Verification items for the finished model (mm, model axes). A direction names the side the tool comes from. Coordinates: 2 decimals unless noted, no trailing zeros. Order: outer loops, then holes, each group sorted by start corner. A loop starts at its lowest first (then second) coordinate and runs counter-clockwise, first axis right, second up. Notation, with made-up numbers: M -21.5,-10 L -9.5,-10 A24 cw -9.5,7 Z; hole C -30,64 d9. An arc over 180 degrees is marked long. Return JSON: item names as keys, results as strings. Group by question number.
Q1. Go/stop test with flat-tipped pins: pin 1 Ø6 at (x, z) = (4, 2.5) entering from -Y; pin 2 Ø6 at (y, z) = (68, -0.5) entering from +X (3 decimals); pin 3 Ø4 at (x, y) = (-4.5, 101) entering from +Z; pin 4 Ø2 at (y, z) = (44, 3.5) entering from +X. Record where each tip stops, or that it passes through.
Q2. Thickness scan on probe 1 along Y at (x, z) = (4.5, 1.5); probe 2 along Z at (x, y) = (0.25, 40). Record the ranges inside material, lowest first.
Q3. Section check A-A, the plane x = 0. Enter the section's corners in (y, z) (3 decimals), then the cut area to 3 significant figures.
Q4. Section check B-B, the plane y = 171. Enter the section's corners in (x, z) (3 decimals), then the cut area to 3 significant figures.
Q5. Access from +Z, -Z, +X, -X, +Y, -Y to the whole of each face (thin tool, end or side, straight path). Record for faces 1 (the face through (0, 2, 5.556)), 2 (the face through (3, 4.366, -3)).
from build123d import *

# Parameters (mm, degrees)
BOSS_EXTRUDE1_DEPTH = 4.365625
SKETCH2_R           = 3.175
BOSS_EXTRUDE2_DEPTH = 177.8


with BuildPart() as part:
    # Sketch1 → Boss-Extrude1 (new body)
    with BuildSketch(Plane(origin=(0, 0, 0), x_dir=(1, 0, 0), z_dir=(0, 1, 0))):
        Polygon((6.415804866, 0), (3.207902433, 5.55625), (-3.207902433, 5.55625), (-6.415804866, 0), (-3.207902433, -5.55625), (3.207902433, -5.55625), align=None)
    extrude(amount=BOSS_EXTRUDE1_DEPTH)

    # Sketch2 → Boss-Extrude2 (add)
    with BuildSketch(Plane(origin=(0, 4.365625, 0), x_dir=(1, 0, 0), z_dir=(0, 1, 0))):
        Circle(SKETCH2_R)
    extrude(amount=BOSS_EXTRUDE2_DEPTH)


solid = part.part
Numbers:
{
 "1": {"pin 1": "stops at y = 0", "pin 2": "stops at x = 3.175", "pin 3": "stops at z = 1.96", "pin 4": "stops at x = 1.96"},
 "2": {"probe 1": "y = 0 to 4.37", "probe 2": "z = -3.17 to 3.17"},
 "3": {"outline": "M 0,-5.556 L 4.366,-5.556 L 4.366,-3.175 L 182.166,-3.175 L 182.166,3.175 L 4.366,3.175 L 4.366,5.556 L 0,5.556 Z", "area": "1,180 mm2"},
 "4": {"outline": "C 0,0 d6.35", "area": "31.7 mm2"},
 "5": {"face 1": "+Z, +X, -X, +Y, -Y", "face 2": "+Y"}
}
